from build123d import *

# Parameters (mm, degrees)
BOSS_EXTRUDE3_DEPTH = 6
BOSS_EXTRUDE5_DEPTH = 50
BOSS_EXTRUDE6_DEPTH = 50
SKETCH4_R           = 6
CUT_EXTRUDE1_DEPTH  = 6
SKETCH5_R           = 6
CUT_EXTRUDE2_DEPTH  = 6


with BuildPart() as part:
    # Sketch1 → Boss-Extrude3 (new body)
    with BuildSketch(Plane(origin=(0, 0, 0), x_dir=(1, 0, 0), z_dir=(0, 1, 0))):
        Polygon((-8.017197152, -238.130630631), (-8.017197152, -204.926643474), (-8.017197152, -63.130630631), (91.982802848, -63.130630631), (91.982802848, -238.130630631), (179.482802848, -238.130630631), (179.482802848, 41.869369369), (-95.517197152, 41.869369369), (-95.517197152, -238.130630631), align=None)
    extrude(amount=BOSS_EXTRUDE3_DEPTH)

    # Sketch2 → Boss-Extrude5 (add)
    with BuildSketch(Plane(origin=(0, 6, 0), x_dir=(1, 0, 0), z_dir=(0, 1, 0))):
        Polygon((-89.517197152, -17.106233318), (-89.517197152, -238.130630631), (-95.517197152, -238.130630631), (-95.517197152, 41.869369369), (-89.517197152, 41.869369369), align=None)
    extrude(amount=BOSS_EXTRUDE5_DEPTH)

    # Sketch3 → Boss-Extrude6 (add)
    with BuildSketch(Plane(origin=(0, 6, 0), x_dir=(1, 0, 0), z_dir=(0, 1, 0))):
        Polygon((173.482802848, -39.36353764), (173.482802848, -238.130630631), (179.482802848, -238.130630631), (179.482802848, 41.869369369), (173.482802848, 41.869369369), align=None)
    extrude(amount=BOSS_EXTRUDE6_DEPTH)

    # Sketch4 → Cut-Extrude1 (cut)
    with BuildSketch(Plane(origin=(179.482802848, 0, 0), x_dir=(0, 0, -1), z_dir=(1, 0, 0))):
        with Locations((-194.630630631, 18.828241407)):
            Circle(SKETCH4_R)
        with Locations((-1.630630631, 18.828241407)):
            Circle(SKETCH4_R)
    extrude(amount=-CUT_EXTRUDE1_DEPTH, mode=Mode.SUBTRACT)

    # Sketch5 → Cut-Extrude2 (cut)
    with BuildSketch(Plane.ZY.offset(95.517197152)):
        with Locations((1.630630631, 18.5)):
            Circle(SKETCH5_R)
        with Locations((194.630630631, 18.5)):
            Circle(SKETCH5_R)
    extrude(amount=-CUT_EXTRUDE2_DEPTH, mode=Mode.SUBTRACT)


solid = part.part
Build history of the part. All positions in model axes, mm. A direction names the side the tool comes from. Coordinates: 2 decimals unless noted, no trailing zeros. Order: outer loops, then holes, each group sorted by start corner. A loop starts at its lowest first (then second) coordinate and runs counter-clockwise, first axis right, second up. Notation, with made-up numbers: M 82,30 L 135,30 A11 cw 135,41 Z; hole C 88.5,-9.75 d7. An arc over 180 degrees is marked long. One line per question, with ' | ' between items. Start each with the question number.
Q1. Saw through at A-A (z = 204). List the corners of the cut face in (x, y), then the cut area to 3 significant figures.
Q2. Saw through at B-B (y = 46). List the corners of the cut face in (x, z), then the cut area to 3 significant figures.
Q3. Probe L1, parallel to X at y = 23.5, z = 28.5; L2, parallel to Y at x = -83, z = 37.5; L3, parallel to X at y = 4.5, z = 124.5. List the from-to ranges inside material, lowest first. Write a range as from..to.
Q4. Flat gauge pins, fed straight in: pin 1 Ø9.5 at (y, z) = (18.5, 194.63) entering from -X; pin 2 Ø12 at (x, z) = (130.5, 72.5) entering from -Y; pin 3 Ø8 at (x, z) = (17, 51) entering from +Y; pin 4 Ø3 at (x, y) = (20, 2) entering from +Z. Where does each tip first touch, or does it go through?
Q5. Saw through at C-C (z = 13.5). List the corners of the cut face in (x, y).
Q6. 3-axis set-ups, long thin cutter, end or side, ignore diameter. For faces 1 (the face through (91.983, 3, 149)), 2 (the face through (-92.559, 18.764, -4.364)), 3 (the face through (176.52, 12.97, 2.93)): which of +Z, -Z, +X, -X, +Y, -Y reach the whole face in a straight line?
Q7. Saw through at D-D (x = 114.5). List the corners of the cut face in (y, z), then the cut area to 3 significant figures.
Q8. Two-plate mould, pull along X, no slides. Class faces 4 (the face through (-95.517, 28, 100)), 5 (the face through (173.483, 31, 96)), 6 (the face through (176, 56, 96)): +X half, -X half, draft (parallel to the pull), parting line (faces both ways), or undercut.
Check values:
1) outline: M -95.52,0 L -8.02,0 L -8.02,6 L -89.52,6 L -89.52,56 L -95.52,56 Z; M 91.98,0 L 179.48,0 L 179.48,56 L 173.48,56 L 173.48,6 L 91.98,6 Z | area: 1,650 mm2
2) outline: M -95.52,-41.87 L -89.52,-41.87 L -89.52,238.13 L -95.52,238.13 Z; M 173.48,-41.87 L 179.48,-41.87 L 179.48,238.13 L 173.48,238.13 Z | area: 3,360 mm2
3) L1: x = -95.52..-89.52, 173.48..179.48 | L2: y = 0..6 | L3: x = -95.52..-8.02, 91.98..179.48
4) pin 1: passes through | pin 2: stops at y = 0 | pin 3: stops at y = 6 | pin 4: stops at z = 63.13
5) outline: M -95.52,0 L 179.48,0 L 179.48,56 L 173.48,56 L 173.48,6 L -89.52,6 L -89.52,56 L -95.52,56 Z
6) face 1: +Z, +Y, -Y | face 2: -X | face 3: +X
7) outline: M 0,-41.87 L 6,-41.87 L 6,238.13 L 0,238.13 Z | area: 1,680 mm2
8) face 4: -X half | face 5: undercut | face 6: draft
